Source: three-view drawing plus pictorial views. Frame: mm from the lowest corner of the part. Give positions to 0.01 mm unless a question says otherwise; leave off trailing zeros. Order: outer loops, then holes, each group sorted by start corner. A loop starts at its lowest first (then second) coordinate and runs counter-clockwise, first axis right, second up. Notation, with made-up numbers: (72.25, 74.5) - (93.25, 74.5) arc R13 cw to (93.25, 88.5) - close; hole circle Ø8 at (3, 45). An arc over 180 degrees is marked (long way). Use one line per item in the form item = value.
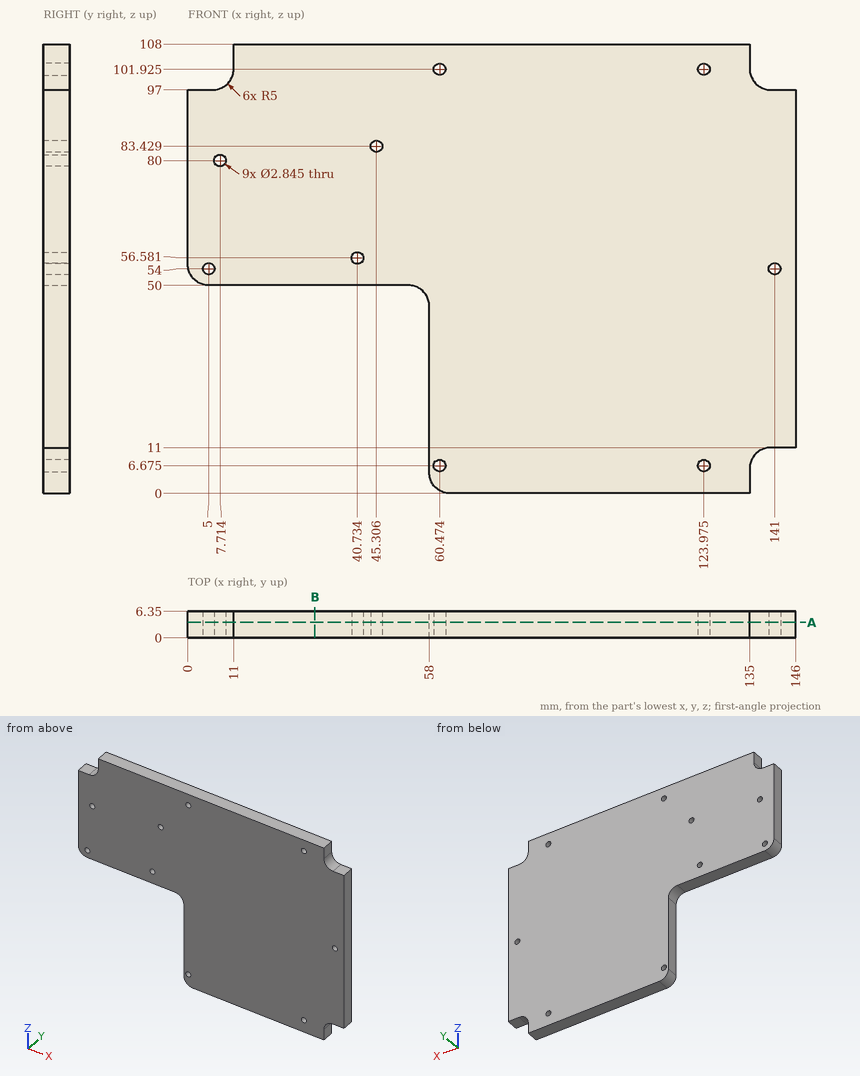
(1) Contact query for flat-ended pins moving along their axis: pin 1 Ø1.8 at (y, z) = (4, 2) entering from +X; pin 2 Ø1.9 at (x, y) = (40, 4.5) entering from -Z; pin 3 Ø3 at (x, y) = (143, 4.5) entering from +Z. Output: stop coordinate, or through.
Computed values:
pin_1 = 135
pin_2 = 50
pin_3 = 97
(2) Cut plane A-A on y = 3.75. Give the number of separate pieces and of enclosed holes in the cut face, plus the area to 3 significant figures.
Computed values:
separate_pieces = 1
enclosed_holes = 9
area = 12,500 mm²
(3) Cut plane B-B on x = 30.5. Output: boundary loops of the cut face in (y, z), plus the area to 3 significant figures.
Computed values:
outline = (0, 50) - (6.35, 50) - (6.35, 108) - (0, 108) - close
area = 368 mm²
(4) Ray query, line 1 along Z through (x, y) = (141, 2); line 2 along X through (y, z) = (4, 80); line 3 along Z through (x, y) = (5, 4.5). Return the intervals inside material, ascending.
Computed values:
line_1 = 11 to 52.58, 55.42 to 97
line_2 = 0 to 6.29, 9.14 to 146
line_3 = 50 to 52.58, 55.42 to 97
